Read the model definition and answer for the solid it produces. Units are mm, in the model's axes. A direction names the side the tool comes from. Round coordinates to 2 decimals unless told otherwise and drop trailing zeros. Loops run counter-clockwise (first coordinate to the right, second up) from the corner with the lowest first, then second, coordinate; pieces in that order, holes last. Notation, with made-up numbers: (-35, -10.5) -> (-14, -10.5) arc R19 cw to (-14, 19.5) -> close; hole circle Ø9 at (62, 43.25). An arc over 180 degrees is marked (long way). Put each result on its own line as item: value.
from build123d import *

# Parameters (mm, degrees)
SKETCH1_W           = 80
SKETCH1_H           = 50
BOSS_EXTRUDE1_DEPTH = 50
CUT_EXTRUDE1_DEPTH  = 30
SKETCH3_W           = 20
SKETCH3_H           = 40
CUT_EXTRUDE2_DEPTH  = 103
CUT_EXTRUDE3_DEPTH  = 103
SKETCH5_W           = 30
SKETCH5_H           = 20
CUT_EXTRUDE4_DEPTH  = 103
CUT_EXTRUDE6_DEPTH  = 103
BOSS_EXTRUDE2_DEPTH = 15
BOSS_EXTRUDE3_DEPTH = 15
SKETCH10_W          = 83.848824186
SKETCH10_H          = 50
CUT_EXTRUDE7_DEPTH  = 15
BOSS_EXTRUDE6_DEPTH = 37


with BuildPart() as part:
    # Sketch1 → Boss-Extrude1 (new body)
    with BuildSketch(Plane.XY):
        with Locations((40, 25)):
            Rectangle(SKETCH1_W, SKETCH1_H)
    extrude(amount=-BOSS_EXTRUDE1_DEPTH)

    # Sketch2 → Cut-Extrude1 (cut)
    with BuildSketch(Plane.XY):
        Polygon((60, 40), (60, 50), (40, 50), (40, 30), align=None)
    extrude(amount=-CUT_EXTRUDE1_DEPTH, mode=Mode.SUBTRACT)

    # Sketch3 → Cut-Extrude2 (cut)
    with BuildSketch(Plane(origin=(0, 0, -50), x_dir=(-1, 0, 0), z_dir=(0, 0, -1))):
        with Locations((-10, 30)):
            Rectangle(SKETCH3_W, SKETCH3_H)
    extrude(amount=-CUT_EXTRUDE2_DEPTH, mode=Mode.SUBTRACT)

    # Sketch4 → Cut-Extrude3 (cut)
    with BuildSketch(Plane(origin=(0, 0, 0), x_dir=(-1, 0, 0), z_dir=(0, -1, 0))):
        Polygon((0, 0), (0, 20), (-40, 0), align=None)
    extrude(amount=-CUT_EXTRUDE3_DEPTH, mode=Mode.SUBTRACT)

    # Sketch5 → Cut-Extrude4 (cut)
    with BuildSketch(Plane(origin=(40, 0, 0), x_dir=(0, 0, -1), z_dir=(1, 0, 0))):
        with Locations((15, 40)):
            Rectangle(SKETCH5_W, SKETCH5_H)
    extrude(amount=-CUT_EXTRUDE4_DEPTH, mode=Mode.SUBTRACT)

    # Sketch6 → Cut-Extrude6 (cut)
    with BuildSketch(Plane(origin=(-4, 8, 0), x_dir=(-0.894427191, -0.447213595, 0), z_dir=(0.447213595, -0.894427191, 0))):
        Polygon((-71.55417528, 30), (-4.472135955, 35), (0, 0), (-71.55417528, 0), align=None)
    extrude(amount=-CUT_EXTRUDE6_DEPTH, mode=Mode.SUBTRACT)

    # Sketch7 → Boss-Extrude2 (add)
    with BuildSketch(Plane(origin=(-4, 8, 0), x_dir=(-0.894427191, -0.447213595, 0), z_dir=(0.447213595, -0.894427191, 0))):
        Polygon((-26.83281573, 33.333333333), (-4.472135955, 50), (-4.472135955, 20), (-26.83281573, 10), align=None)
        Polygon((-26.83281573, 50), (-4.472135955, 50), (-26.83281573, 33.333333333), align=None)
    extrude(amount=BOSS_EXTRUDE2_DEPTH)

    # Sketch8 → Boss-Extrude3 (add)
    with BuildSketch(Plane(origin=(8, 0, -16), x_dir=(0.894427191, 0, 0.447213595), z_dir=(-0.447213595, 0, 0.894427191))):
        Polygon((13.416407865, 10), (-8.94427191, 10), (13.416407865, 20), align=None)
    extrude(amount=-BOSS_EXTRUDE3_DEPTH)

    # Sketch10 → Cut-Extrude7 (cut)
    with BuildSketch(Plane(origin=(0, 0, 0), x_dir=(-1, 0, 0), z_dir=(0, -1, 0))):
        with Locations((-38.075587907, 25)):
            Rectangle(SKETCH10_W, SKETCH10_H)
    extrude(amount=CUT_EXTRUDE7_DEPTH, mode=Mode.SUBTRACT)

    # Sketch15 → Boss-Extrude6 (add)
    with BuildSketch(Plane(origin=(0, 50, 0), x_dir=(1, 0, 0), z_dir=(0, 1, 0))):
        Polygon((55, 30), (60, 30), (62.90753881, 30), (62.90753881, 35.567139934), (20, 35.567139934), (20, 32.333333333), align=None)
        Polygon((20, 30), (55, 30), (20, 32.333333333), align=None)
    extrude(amount=-BOSS_EXTRUDE6_DEPTH)


solid = part.part
Item 1: Which of the six approach directions +Z, -Z, +X, -X, +Y, -Y give full straight-line access (tool end or side, diameter ignored) to faces 1 (the flat face through (80, 25, -25)), 2 (the flat face through (60, 45, -15)), 3 (the flat face through (20, 35, -40))?
Derived:
face 1: +Z, -Z, +X, +Y, -Y
face 2: +Z, -X, +Y
face 3: +Z, -Z, -X, +Y
Item 2: Find the intervals of material crossed by line 1 along X through (y, z) = (45, -33.5); line 2 along X through (y, z) = (30, -7.5); line 3 along Z through (x, y) = (31, 45), in increasing order.
Derived:
line 1: x = 20 to 80
line 2: x = 40 to 80
line 3: z = -50 to -30
Item 3: The part is cut by section B-B (y = 41.5). Determine the outline of the cut face in (x, z), then the cut area to 3 significant figures.
Derived:
outline: (20, -50) -> (80, -50) -> (80, 0) -> (60, 0) -> (60, -30) -> (20, -30) -> close
area: 1,800 mm^2
Item 4: Flat-ended cylindrical pins translate along their axes: pin 1 Ø2 at (x, y) = (25.5, 27) entering from +Z; pin 2 Ø1 at (x, z) = (22, -28) entering from +Y; pin 3 Ø5 at (y, z) = (46.5, -14.5) entering from -X. Find the tip coordinate at first contact, or state that the pin passes through.
Derived:
pin 1: stops at z = -30
pin 2: stops at y = 21.25
pin 3: stops at x = 60
Item 5: The part is cut by section D-D (z = -16). Determine the outline of the cut face in (x, y), then the cut area to 3 significant figures.
Derived:
outline: (8, 0) -> (80, 0) -> (80, 50) -> (60, 50) -> (60, 40) -> (8, 14) -> close
area: 2,400 mm^2
Item 6: The part is cut by section C-C (x = 10). Determine the outline of the cut face in (y, z).
Derived:
outline: (0, -50) -> (15, -50) -> (15, -15) -> (0, -15) -> close
Item 7: The part is cut by section A-A (z = -28). Determine the outline of the cut face in (x, y), then the cut area to 3 significant figures.
Derived:
outline: (0, 0) -> (80, 0) -> (80, 50) -> (60, 50) -> (60, 40) -> (0, 10) -> close
area: 2,500 mm^2
